Read the model definition and answer for the solid it produces. Units are mm, in the model's axes. Round coordinates to 2 decimals unless told otherwise and drop trailing zeros. Write each loop counter-clockwise with the first axis right and the second up, starting at its lowest first coordinate (ties: lowest second). Pieces come first, ordered by that corner, then holes. Notation, with made-up numbers: (-31, 1.5) -> (5, 1.5) arc R18 ccw to (5, 33.5) -> close; hole circle Ø9 at (66.25, 78). An arc over 180 degrees is marked (long way). Return JSON: item names as keys, results as strings. Group by question number.
(1) A cutting plane is placed at A-A on y = 0. Give the vertices of the cut face in (x, z).
(2) A cutting plane is placed at D-D on z = 4. State how many separate pieces and enclosed holes the cut face has, then the cut area to 3 significant figures.
(3) Straight lines are drawn through the part: line 1 (X direction, y = 60.5, z = 2); line 2 (Y direction, x = -39.37, z = 3.75); line 3 (Y direction, x = 39, z = 0.5). For each, find the intervals that lie inside material, in ascending order.
(4) A cutting plane is placed at C-C on x = 25.4. Give the vertices of the cut face in (y, z), then the cut area to 3 significant figures.
(5) A cutting plane is placed at B-B on x = 39.37. Give the vertices of the cut face in (y, z), then the cut area to 3 significant figures.
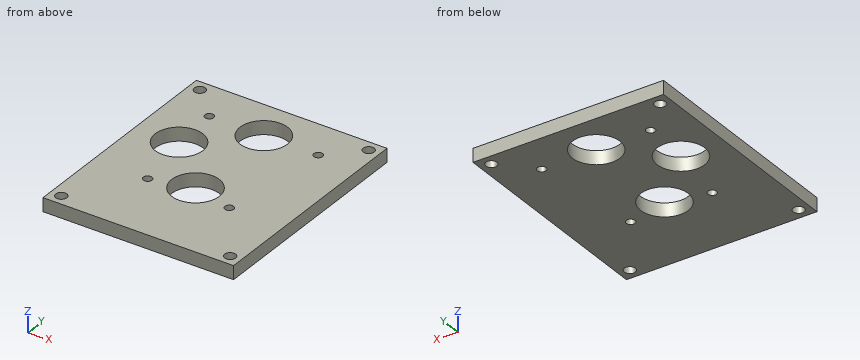
Autodesk Inventor part; units mm, degrees
ref_plane "YZ Plane" through (0, 0, 0) normal (1, 0, 0) x (0, 1, 0)
ref_plane "XZ Plane" through (0, 0, 0) normal (0, 1, 0) x (-1, 0, 0)
ref_plane "XY Plane" through (0, 0, 0) normal (0, 0, 1) x (1, 0, 0)
sketch "Sketch1" plane through (0, 0, 0) normal (0, 0, 1) x (1, 0, 0)
  circle A0 centre (0, 0) radius 11.1125
  line L0 (0, 0) -> (-24.2467, 24.2467) construction
  line L1 (0, 0) -> (34.29, 0) construction
  circle A1 centre (-24.2467, 24.2467) radius 11.1125
  line L2 (-24.2467, 24.2467) -> (8.7733, 24.2467) construction
  line L3 (-24.2467, 24.2467) -> (0, 24.2467) construction
  line L4 (0, 24.2467) -> (0, 46.6502) construction
  line L5 (0, 46.6502) -> (-24.2467, 24.2467) construction
  circle A2 centre (0, 46.6502) radius 11.1125
  line L6 (0, 46.6502) -> (-25.4, 46.6502) construction
  line L7 (-25.4, 46.6502) -> (25.4, 46.6502) construction
  circle A3 centre (-25.4, 46.6502) radius 2.032
  circle A4 centre (25.4, 46.6502) radius 2.032
  line L8 (0, 46.6502) -> (0, 65.7002) construction
  line L9 (0, 65.7002) -> (44.45, 65.7002)
  line L10 (44.45, 65.7002) -> (44.45, -39.0748)
  line L11 (0, 65.7002) -> (-44.45, 65.7002)
  line L12 (-44.45, 65.7002) -> (-44.45, -39.0748)
  line L13 (-44.45, -39.0748) -> (44.45, -39.0748)
  dimension "d0" = 22.225
  dimension "d1" = 34.29
  dimension "d2" = 135
  dimension "d3" = 22.225
  dimension "d7" = 22.4035
  dimension "d8" = 22.225
  dimension "d9" = 25.4
  dimension "d10" = 50.8
  dimension "d11" = 4.064
  dimension "d12" = 19.05
  dimension "d13" = 104.775
  dimension "d14" = 44.45
  dimension "d17" = 44.45
extrude "Extrusion1" add sketch "Sketch1" along normal blind 6.35
sketch "Sketch2" plane through (0, 0, 6.35) normal (0, 0, 1) x (1, 0, 0)
  line L0 (-44.45, 65.7002) -> (-39.37, 65.7002) construction
  line L1 (-44.45, 65.7002) -> (44.45, 65.7002) construction
  line L2 (-39.37, 65.7002) -> (-39.37, 60.6202) construction
  circle A0 centre (-39.37, 60.6202) radius 2.5797
  line L3 (0, 65.7002) -> (0, -39.0748) construction
  line L4 (-44.45, -39.0748) -> (44.45, -39.0748) construction
  line L5 (44.45, -39.0748) -> (44.45, 65.7002) construction
  line L6 (44.45, 13.3127) -> (-44.45, 13.3127) construction
  circle A1 centre (39.37, 60.6202) radius 2.5797
  circle A2 centre (-39.37, -33.9948) radius 2.5797
  circle A3 centre (39.37, -33.9948) radius 2.5797
  point P0 (0, 0)
  dimension "d18" = 5.08
  dimension "d19" = 5.08
  dimension "d20" = 5.1594
extrude "Extrusion2" cut sketch "Sketch2" against normal blind 25.4
sketch "Sketch3" plane through (0, 0, 6.35) normal (0, 0, 1) x (1, 0, 0)
  line L0 (0, 0) -> (19.05, 0) construction
  line L1 (19.05, 0) -> (19.05, -4.7752) construction
  line L2 (0, 0) -> (0, -18.8827) construction
  circle A0 centre (19.05, -4.7752) radius 2.0193
  circle A1 centre (-19.05, -4.7752) radius 2.0193
  dimension "d23" = 19.05
  dimension "d24" = 4.7752
  dimension "d25" = 4.0386
extrude "Extrusion3" cut sketch "Sketch3" against normal blind 25.4
properties part number "Gearbox Plate V2"
Checks:
{
 "1": {"outline": "(-44.45, 0) -> (-11.11, 0) -> (-11.11, 6.35) -> (-44.45, 6.35) -> close; (11.11, 0) -> (44.45, 0) -> (44.45, 6.35) -> (11.11, 6.35) -> close"},
 "2": {"separate pieces": "1", "enclosed holes": "11", "area": "8,020 mm^2"},
 "3": {"line 1": "x = -44.45 to -41.95, -36.79 to 36.79, 41.95 to 44.45", "line 2": "y = -39.07 to -36.57, -31.42 to 58.04, 63.2 to 65.7", "line 3": "y = -39.07 to -36.55, -31.44 to 58.07, 63.17 to 65.7"},
 "4": {"outline": "(-39.07, 0) -> (44.62, 0) -> (44.62, 6.35) -> (-39.07, 6.35) -> close; (48.68, 0) -> (65.7, 0) -> (65.7, 6.35) -> (48.68, 6.35) -> close", "area": "640 mm^2"},
 "5": {"outline": "(-39.07, 0) -> (-36.57, 0) -> (-36.57, 6.35) -> (-39.07, 6.35) -> close; (-31.42, 0) -> (58.04, 0) -> (58.04, 6.35) -> (-31.42, 6.35) -> close; (63.2, 0) -> (65.7, 0) -> (65.7, 6.35) -> (63.2, 6.35) -> close", "area": "600 mm^2"}
}
